Autodesk Inventor part; units mm, degrees
ref_plane "Work Plane1" through (-2.5, 3, 0) normal (0, 1, 0) x (1, 0, 0)
ref_plane "YZ Plane" through (0, 0, 0) normal (1, 0, 0) x (0, 1, 0)
ref_plane "XZ Plane" through (0, 0, 0) normal (0, 1, 0) x (-1, 0, 0)
ref_plane "Work Plane1" through (-2.5, 3, 0) normal (0, 1, 0) x (1, 0, 0)
sketch "草圖8" plane through (-2.5, 3, 0) normal (0, 1, 0) x (1, 0, 0)
  circle A0 centre (2.5, -1.5) radius 5
  point P0 (2.5, 0)
  point P1 (2.5, 0)
  dimension "d26" = 10
extrude "擠出6" add sketch "草圖8" along normal blind 3
sketch "草圖9" plane through (0, 6, 1.5) normal (0, 1, 0) x (1, 0, 0)
  circle A0 centre (0, 0) radius 1.5
  point P0 (0, 1.5)
  dimension "d29" = 3
extrude "擠出7" add sketch "草圖9" along normal blind 35
sketch "Sketch10" plane through (0, 3, 1.5) normal (0, -1, 0) x (1, 0, 0)
  line L0 (0, 0) -> (0, 3) construction
  circle A0 centre (0, 0) radius 5
  line L1 (0, 3) -> (-4, 3)
  line L2 (0, 3) -> (4, 3)
  line L3 (0, 0) -> (0, -3) construction
  line L4 (0, -3) -> (-4, -3)
  line L5 (0, -3) -> (4, -3)
  point P0 (0, -1.5)
  dimension "d34" = 3
  dimension "d35" = 3
extrude "Extrusion8" add sketch "Sketch10" along normal blind 7 contours A0 L5 L4 L1 L2
sketch "Sketch11" plane through (-4, 3, 4.5) normal (0, 0, 1) x (1, 0, 0)
  line L0 (0, 0) -> (8, 0) construction
  line L1 (4, 0) -> (4, -3.5) construction
  circle A0 centre (4, -3.5) radius 1.8
  line L2 (-1, -7) -> (-1, 3) construction
  line L3 (-1, 0) -> (-1, -5) construction
  line L4 (9, -7) -> (9, 3) construction
  line L5 (9, 0) -> (9, -5) construction
  arc A1 (-1, -5) -> (9, -5) centre (4, 0) ccw
  line L6 (-1, -7) -> (0, -7)
  line L7 (-1, -5) -> (-1, -7)
  line L8 (8, -7) -> (9, -7)
  line L9 (9, -7) -> (9, -5)
  line L10 (-1, -7) -> (3, -7)
  line L11 (8, -7) -> (0, -7)
  line L12 (9, -7) -> (5, -7)
  point P0 (4, -3)
  dimension "d38" = 3.5
  dimension "d39" = 3.6
  dimension "d40" = 5
extrude "Extrusion9" cut sketch "Sketch11" against normal through all contours A0
extrude "Extrusion10" cut sketch "Sketch11" against normal blind 7 contours A1 L9 L8 L11 | A1 L10 L6 L7
equation "\"d41\" = d38"
properties part number "避震"
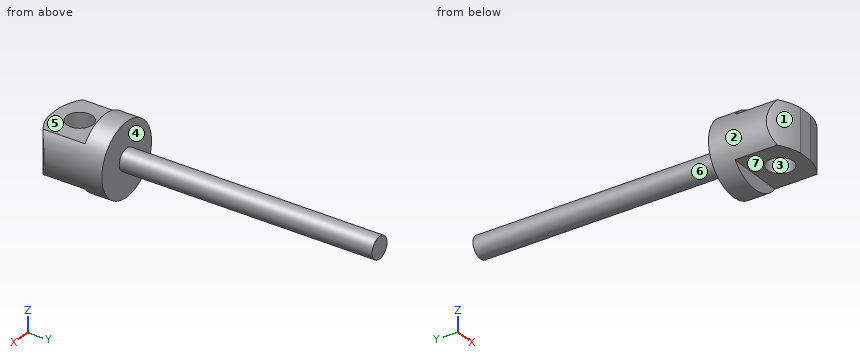
Could you check a few things on this model? Use its own coordinates, in mm. Face numbers are marked on the shaded views. A direction names the side the tool comes from. Coordinates: 2 decimals unless noted, no trailing zeros. Loops run counter-clockwise (first coordinate to the right, second up) from the corner with the lowest first, then second, coordinate; pieces in that order, holes last.
1. For P1, Ø6, axis at x = -3, y = 11.5, coming from the -Z side; P2, Ø1, axis at x = -1, z = -2.5, coming from the -Y side; P3, Ø2, axis at x = 1, y = -0.5, coming from the +Z side, each with a flat end and sliding along its axis, tell me the tip position at first contact or that it passes through.
2. Imagine slicing it at B-B (x = 0). Please give me the cut outline in (y, z), and give its area (3 significant figures).
3. Imagine slicing it at D-D (x = 3). Please give me the cut outline in (y, z).
4. I need wall thicknesses on L1, parallel to Y at x = 0, z = 0.7; L2, parallel to Y at x = 0, z = 3.05; L3, parallel to Y at x = -2.25, z = 5. Which ranges of each line are inside material? Lowest first, please.
5. Imagine slicing it at A-A (y = -0.5). Please give me the cut outline in (x, z), and give its area (3 significant figures).
6. For the marked faces 5, 6 and 7, which set-ups out of +Z, -Z, +X, -X, +Y, -Y let a thin tool reach every point of the face, with its end or its side?
7. We'd pull the mould along X, two halves only. Please class the marked faces 1, 2, 3 and 4: released by +X, released by -X, zero draft, split by the parting line, or undercut.
8. Imagine slicing it at C-C (z = 1.5). Please give me the cut outline in (x, y).
Computed values:
1. P1: stops at z = 0
1. P2: stops at y = 3
1. P3: stops at z = 4.5
2. outline: (-4, -1.5) - (-2.3, -1.5) - (-2.3, 4.5) - (-4, 4.5) - close; (1.3, -1.5) - (3, -1.5) - (3, -3.5) - (6, -3.5) - (6, 0) - (41, 0) - (41, 3) - (6, 3) - (6, 6.5) - (3, 6.5) - (3, 4.5) - (1.3, 4.5) - close
2. area: 155 mm2
3. outline: (-3.4, -1.5) - (3, -1.5) - (3, -2.5) - (6, -2.5) - (6, 5.5) - (3, 5.5) - (3, 4.5) - (-3.4, 4.5) - close
4. L1: y = -4 to -2.3, 1.3 to 41
4. L2: y = -4 to -2.3, 1.3 to 6
4. L3: y = 3 to 6
5. outline: (-4, -1.5) - (-1.8, -1.5) - (-1.8, 4.5) - (-4, 4.5) arc R5 ccw to start; (1.8, -1.5) - (4, -1.5) arc R5 ccw to (4, 4.5) - (1.8, 4.5) - close
5. area: 34.6 mm2
6. face 5: +Z, +X, -X, -Y
6. face 6: +Y
6. face 7: -Z, +X, -X, -Y
7. face 1: released by -X
7. face 2: split by the parting line
7. face 3: undercut
7. face 4: zero draft
8. outline: (-5, -2) arc R7.07 ccw to (-1, -4) - (1, -4) arc R7.07 ccw to (5, -2) - (5, 6) - (1.5, 6) - (1.5, 41) - (-1.5, 41) - (-1.5, 6) - (-5, 6) - close; hole circle Ø3.6 at (0, -0.5)
